Work out the finished part from the listing and answer in its coordinate system (mm). Face numbers are marked on the shaded views. A direction names the side the tool comes from. Give positions to 0.01 mm unless a question says otherwise; leave off trailing zeros. Loops run counter-clockwise (first coordinate to the right, second up) from the corner with the lowest first, then second, coordinate; pieces in that order, holes last. Notation, with made-up numbers: M 45.5,80.25 L 102.5,80.25 A5 ccw 102.5,84.25 Z; hole C -39,6 d1. An arc over 180 degrees is marked long. Answer as a JSON object with one key per item and string values. Group by question number.
```python
from build123d import *

# Parameters (mm, degrees)
SKETCH1_W           = 60
SKETCH1_H           = 30
BOSS_EXTRUDE1_DEPTH = 4
SKETCH2_W           = 8.7752
SKETCH2_H           = 17.5504
SKETCH2_R           = 1.1
BOSS_EXTRUDE2_DEPTH = 4
CHAMFER1_SIZE       = 6.2
CHAMFER1_SIZE_2     = 4.026327078


with BuildPart() as part:
    # Sketch1 → Boss-Extrude1 (new body)
    with BuildSketch(Plane(origin=(0, 0, 0), x_dir=(1, 0, 0), z_dir=(0, 1, 0))):
        Rectangle(SKETCH1_W, SKETCH1_H)
    extrude(amount=BOSS_EXTRUDE1_DEPTH)

    # Sketch2 → Boss-Extrude2 (add)
    # profile 1 of 4: a face of its own
    with BuildSketch(Plane(origin=(0, 4, 0), x_dir=(1, 0, 0), z_dir=(0, 1, 0))):
        with Locations((-25.6124, 15)):
            Rectangle(SKETCH2_W, SKETCH2_H)
        with Locations(Location((-25.6124, 19.3876, 0), (0, 0, 270))):
            Circle(SKETCH2_R, mode=Mode.SUBTRACT)
    # profile 2 of 4: a face of its own
    with BuildSketch(Plane(origin=(0, 4, 0), x_dir=(1, 0, 0), z_dir=(0, 1, 0))):
        with Locations((-25.6124, -15)):
            Rectangle(SKETCH2_W, SKETCH2_H)
        with Locations(Location((-25.6124, -19.3876, 0), (0, 0, 90))):
            Circle(SKETCH2_R, mode=Mode.SUBTRACT)
    # profile 3 of 4: a face of its own
    with BuildSketch(Plane(origin=(0, 4, 0), x_dir=(1, 0, 0), z_dir=(0, 1, 0))):
        with Locations((25.6124, -15)):
            Rectangle(SKETCH2_W, SKETCH2_H)
        with Locations(Location((25.6124, -19.3876, 0), (0, 0, 270))):
            Circle(SKETCH2_R, mode=Mode.SUBTRACT)
    # profile 4 of 4: a face of its own
    with BuildSketch(Plane(origin=(0, 4, 0), x_dir=(1, 0, 0), z_dir=(0, 1, 0))):
        with Locations((25.6124, 15)):
            Rectangle(SKETCH2_W, SKETCH2_H)
        with Locations(Location((25.6124, 19.3876, 0), (0, 0, 90))):
            Circle(SKETCH2_R, mode=Mode.SUBTRACT)
    extrude(amount=BOSS_EXTRUDE2_DEPTH)

    # Chamfer1
    # the kernel refuses this chamfer: 6.2, 4.026327078 mm, written as the material it adds along each edge
    with BuildSketch(Plane(origin=(30, 4, -6.2248), x_dir=(0, -0.021073765466273358, 0.9997779235455605), z_dir=(-1, 0, 0))) as chamfer1_piece_1_section:
        Polygon((CHAMFER1_SIZE * 0.999777923546, CHAMFER1_SIZE * 0.0210737654663), (-CHAMFER1_SIZE_2 * 0.0210737654654, CHAMFER1_SIZE_2 * 0.999777923502), (0, 0), align=None)
    chamfer1_piece_1 = extrude(amount=8.7752, mode=Mode.PRIVATE)
    chamfer1_piece_1 = split(chamfer1_piece_1, bisect_by=Plane(origin=(25.6124, 8, -4.147892519), z_dir=(0, -1, 0)), keep=Keep.TOP, mode=Mode.PRIVATE)
    add(chamfer1_piece_1)
    with BuildSketch(Plane(origin=(30, 4, 6.2248), x_dir=(0, -0.021073765466273358, -0.9997779235455605), z_dir=(-1, 0, 0))) as chamfer1_piece_2_section:
        Polygon((CHAMFER1_SIZE * 0.999777923546, -CHAMFER1_SIZE * 0.0210737654663), (-CHAMFER1_SIZE_2 * 0.0210737654654, -CHAMFER1_SIZE_2 * 0.999777923502), (0, 0), align=None)
    chamfer1_piece_2 = extrude(amount=8.7752, mode=Mode.PRIVATE)
    chamfer1_piece_2 = split(chamfer1_piece_2, bisect_by=Plane(origin=(25.6124, 8, 4.147892519), z_dir=(0, -1, 0)), keep=Keep.TOP, mode=Mode.PRIVATE)
    add(chamfer1_piece_2)
    with BuildSketch(Plane(origin=(-30, 4, 6.2248), x_dir=(0, -0.021073765466273358, -0.9997779235455605), z_dir=(1, 0, 0))) as chamfer1_piece_3_section:
        Polygon((CHAMFER1_SIZE * 0.999777923546, CHAMFER1_SIZE * 0.0210737654663), (-CHAMFER1_SIZE_2 * 0.0210737654654, CHAMFER1_SIZE_2 * 0.999777923502), (0, 0), align=None)
    chamfer1_piece_3 = extrude(amount=8.7752, mode=Mode.PRIVATE)
    chamfer1_piece_3 = split(chamfer1_piece_3, bisect_by=Plane(origin=(-25.6124, 8, 4.147892519), z_dir=(0, -1, 0)), keep=Keep.TOP, mode=Mode.PRIVATE)
    add(chamfer1_piece_3)
    with BuildSketch(Plane(origin=(-30, 4, -6.2248), x_dir=(0, -0.021073765466273358, 0.9997779235455605), z_dir=(1, 0, 0))) as chamfer1_piece_4_section:
        Polygon((CHAMFER1_SIZE * 0.999777923546, -CHAMFER1_SIZE * 0.0210737654663), (-CHAMFER1_SIZE_2 * 0.0210737654654, -CHAMFER1_SIZE_2 * 0.999777923502), (0, 0), align=None)
    chamfer1_piece_4 = extrude(amount=8.7752, mode=Mode.PRIVATE)
    chamfer1_piece_4 = split(chamfer1_piece_4, bisect_by=Plane(origin=(-25.6124, 8, -4.147892519), z_dir=(0, -1, 0)), keep=Keep.TOP, mode=Mode.PRIVATE)
    add(chamfer1_piece_4)


solid = part.part
```
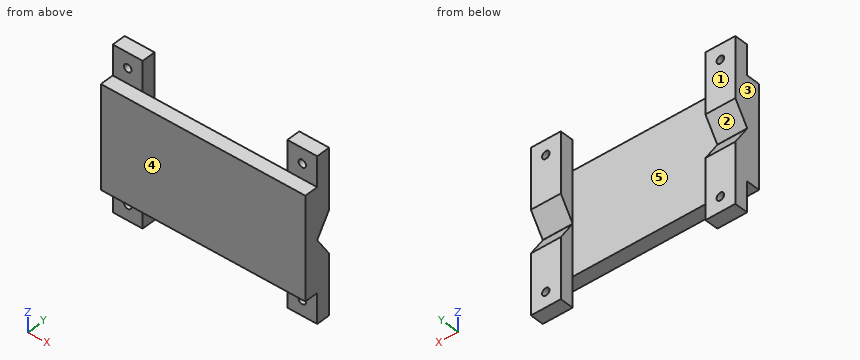
Item 1: Find the intervals of material crossed by probe 1 along X at (y, z) = (6.5, -18.5); probe 2 along X at (y, z) = (6, -13); probe 3 along Z at (x, y) = (-6.5, 1.5), in increasing order. Write a range as [from, to].
Item 2: Given pin 1 Ø1.2 at (x, y) = (13, 1.5) entering from -Z; pin 2 Ø15 at (x, z) = (2, 1) entering from +Y; pin 3 Ø1.5 at (x, y) = (8, 4.5) entering from +Z, each flat-ended and moving along its own axis, determine where each tip first touches the part or whether it passes through.
Item 3: For a pull along X with two mould halves and no side action, classify the marked faces 3, 4 and 5 as pulls with the +X half, pulls with the -X half, needs draft (parallel to the pull), parting line crosses it, or undercut.
Item 4: A cutting plane is placed at A-A (y = 6.25). Determine the outline of the cut face in (x, z).
Item 5: A cutting plane is placed at C-C (x = 7). Determine the outline of the cut face in (y, z), and give its area (3 significant figures).
Item 6: A cutting plane is placed at B-B (z = -9). Determine the outline of the cut face in (x, y), and give its area (3 significant figures).
Item 7: A tool of negligible diameter and unlimited length cuts with its end or side. For the marked faces 1 and 2, from which of +Z, -Z, +X, -X, +Y, -Y can it reach the whole face along a straight path? Write none if from no direction.
Item 8: A cutting plane is placed at D-D (y = 2). Determine the outline of the cut face in (x, z).
The answers:
{
 "1": {"probe 1": "x = [-30, -26.26], [-24.96, -21.22], [21.22, 24.96], [26.26, 30]", "probe 2": "x = [-30, -21.22], [21.22, 30]", "probe 3": "z = [-15, 15]"},
 "2": {"pin 1": "stops at z = -15", "pin 2": "stops at y = 4", "pin 3": "stops at z = 15"},
 "3": {"face 3": "pulls with the -X half", "face 4": "needs draft", "face 5": "undercut"},
 "4": {"outline": "M -30,-23.78 L -21.22,-23.78 L -21.22,-3.49 L -30,-3.49 Z; M -30,3.49 L -21.22,3.49 L -21.22,23.78 L -30,23.78 Z; M 21.22,-23.78 L 30,-23.78 L 30,-3.49 L 21.22,-3.49 Z; M 21.22,3.49 L 30,3.49 L 30,23.78 L 21.22,23.78 Z; hole C -25.61,-19.39 d2.2; hole C -25.61,19.39 d2.2; hole C 25.61,-19.39 d2.2; hole C 25.61,19.39 d2.2"},
 "5": {"outline": "M 0,-15 L 4,-15 L 4,15 L 0,15 Z", "area": "120 mm^2"},
 "6": {"outline": "M -30,0 L 30,0 L 30,8 L 21.22,8 L 21.22,4 L -21.22,4 L -21.22,8 L -30,8 Z", "area": "310 mm^2"},
 "7": {"face 1": "+Z, -Z, +X, -X, +Y", "face 2": "+X, -X, +Y"},
 "8": {"outline": "M -30,-15 L 30,-15 L 30,15 L -30,15 Z"}
}
